```python
from build123d import *
from build123d.topology import SkipClean

# Parameters (mm, degrees)
SKETCH_1_R      = 20
SKETCH_1_R_2    = 5
EXTRUDE_1_DEPTH = 16
EXTRUDE_START   = 3
SKETCH_2_R      = 24
SKETCH_2_R_2    = 5
EXTRUDE_2_DEPTH = 3
EXTRUDE_START_2 = -16
SKETCH_2_2_R    = 24
SKETCH_2_2_R_2  = 5
EXTRUDE_3_DEPTH = 3


with BuildPart() as part:
    # 草图1 → 凸台-拉伸1 (new body)
    with BuildSketch(Plane(origin=(0, 0, 0), x_dir=(1, 0, 0), z_dir=(0, 1, 0))):
        with Locations(Location((0, 0, 0), (0, 0, 270))):
            Circle(SKETCH_1_R)
        with Locations(Location((0, 0, 0), (0, 0, 270))):
            Circle(SKETCH_1_R_2, mode=Mode.SUBTRACT)
    extrude(amount=EXTRUDE_1_DEPTH)

    # 草图2 → 凸台-拉伸2 (add)
    with SkipClean():  # the faces are left unmerged after this step: merging them gives an invalid solid
        with BuildSketch(Plane.XZ.offset(EXTRUDE_START)):
            with Locations(Location((0, 0, 0), (0, 0, 270))):
                Circle(SKETCH_2_R)
            with Locations(Location((0, 0, 0), (0, 0, 270))):
                Circle(SKETCH_2_R_2, mode=Mode.SUBTRACT)
        extrude(amount=-EXTRUDE_2_DEPTH)

    # 草图2<2> → 凸台-拉伸3 (add)
    with BuildSketch(Plane.XZ.offset(EXTRUDE_START_2)):
        with Locations(Location((0, 0, 0), (0, 0, 270))):
            Circle(SKETCH_2_2_R)
        with Locations(Location((0, 0, 0), (0, 0, 270))):
            Circle(SKETCH_2_2_R_2, mode=Mode.SUBTRACT)
    extrude(amount=-EXTRUDE_3_DEPTH)


solid = part.part
```
Here's how the part is built. I have some questions about the finished solid (model axes, mm). A direction names the side the tool comes from. Round coordinates to 2 decimals unless told otherwise and drop trailing zeros. Write each loop counter-clockwise with the first axis right and the second up, starting at its lowest first coordinate (ties: lowest second). Pieces come first, ordered by that corner, then holes.
Q1. If we section it at C-C on y = 9.5: Write out the boundary of the cut face in (x, z), plus the area to 3 significant figures.
Q2. If we section it at D-D on z = 16: Write out the boundary of the cut face in (x, y).
Q3. Which directions (+Z, -Z, +X, -X, +Y, -Y) give clear straight access to the entire face, cutting with the end or side of a thin tool? Please do faces 4 (the cylindrical face through (7.21, 17.48, -22.89)), 5 (the flat face through (20, 16, 5)).
Q4. If we mould it in two halves opening along Y, with no side actions, what happens to faces 1 (the cylindrical face through (-19.524, 7.888, -4.336)), 2 (the flat face through (6, -3, 0)), 3 (the flat face through (6, 19, 0))? For each: +Y half, -Y half, draft (parallel to the pull), parting line (faces both ways), or undercut.
Q5. Will these pins go through, and if not, where does the flat tip stop? P1, Ø11.5, axis at x = 0, z = 0, coming from the -Y side; P2, Ø1, axis at x = -16, y = 6, coming from the +Z side; P3, Ø10, axis at y = 16.5, z = -7.5, coming from the +X side; P4, Ø1.5, axis at x = -6, y = 1.5, coming from the +Z side.
Q6. If we section it at B-B on x = 0: Write out the boundary of the cut face in (y, z).
Q7. If we section it at A-A on z = 0: Write out the boundary of the cut face in (x, y), plus the area to 3 significant figures.
Q8. Please list where these lines run through material, in increasing order: probe 1 along X at (y, z) = (7.5, 0); probe 2 along X at (y, z) = (17.8, 0); probe 3 along Y at (x, z) = (10, -19).
Answer below:
1. outline: circle Ø40 at (0, 0); hole circle Ø10 at (0, 0)
1. area: 1,180 mm2
2. outline: (-17.89, -3) - (17.89, -3) - (17.89, 0) - (12, 0) - (12, 16) - (17.89, 16) - (17.89, 19) - (-17.89, 19) - (-17.89, 16) - (-12, 16) - (-12, 0) - (-17.89, 0) - close
3. face 4: +Y, -Y
3. face 5: none
4. face 1: undercut
4. face 2: -Y half
4. face 3: +Y half
5. P1: stops at y = -3
5. P2: stops at z = 12.64
5. P3: stops at x = 23.87
5. P4: stops at z = 19.3
6. outline: (-3, -24) - (0, -24) - (0, -20) - (16, -20) - (16, -24) - (19, -24) - (19, -5) - (-3, -5) - close; (-3, 5) - (19, 5) - (19, 24) - (16, 24) - (16, 20) - (0, 20) - (0, 24) - (-3, 24) - close
7. outline: (-24, -3) - (-5, -3) - (-5, 19) - (-24, 19) - (-24, 16) - (-20, 16) - (-20, 0) - (-24, 0) - close; (5, -3) - (24, -3) - (24, 0) - (20, 0) - (20, 16) - (24, 16) - (24, 19) - (5, 19) - close
7. area: 708 mm2
8. probe 1: x = -20 to -5, 5 to 20
8. probe 2: x = -24 to -5, 5 to 24
8. probe 3: y = -3 to 0, 16 to 19
